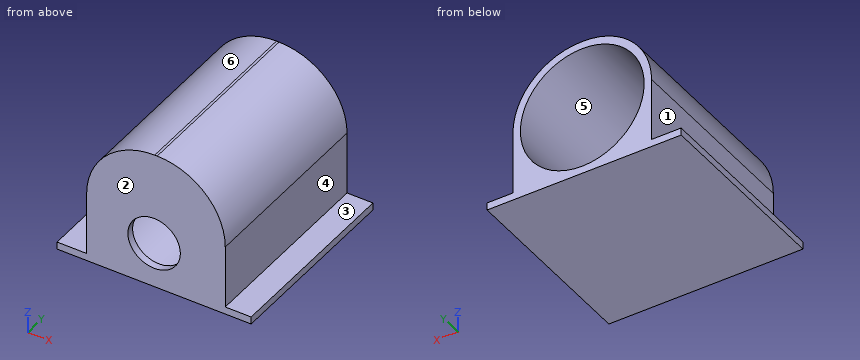
from build123d import *

# Parameters (mm, degrees)
SKETCH018_W     = 52.5
SKETCH018_H     = 2
PAD014_DEPTH    = 51.3
SKETCH028_W     = 37.5
SKETCH028_H     = 51.3
PAD015_DEPTH    = 35.5
FILLET001_R     = 18.416667
SKETCH031_R     = 7.1
POCKET005_DEPTH = 2
SKETCH032_R     = 16.75
POCKET006_DEPTH = 49.3


with BuildPart() as part:
    # Sketch018 → Pad014 (new body)
    with BuildSketch(Plane.XZ):
        with Locations((36.25, 3)):
            Rectangle(SKETCH018_W, SKETCH018_H)
    extrude(amount=-PAD014_DEPTH)

    # Sketch028 (on Face1 of Pad014) → Pad015 (join)
    with BuildSketch(Plane(origin=(0, 0, 4), x_dir=(-1, 0, 0), z_dir=(0, 0, 1))):
        with Locations((-36.75, -25.65)):
            Rectangle(SKETCH028_W, SKETCH028_H)
    extrude(amount=PAD015_DEPTH)

    # Fillet001
    fillet001_edges = [part.edges().sort_by_distance(p)[0] for p in [
        (18, 25.65, 39.5),
        (55.5, 25.65, 39.5),
    ]]
    fillet(fillet001_edges, radius=FILLET001_R)

    # Sketch031 (on Face6 of Pad015) → Pocket005 (cut)
    with BuildSketch(Plane.XZ):
        with Locations((36.25, 14.3)):
            Circle(SKETCH031_R)
    extrude(amount=-POCKET005_DEPTH, mode=Mode.SUBTRACT)

    # Sketch032 (on Face5 of Pocket005) → Pocket006 (cut)
    with BuildSketch(Plane(origin=(0, 51.3, 0), x_dir=(1, 0, 0), z_dir=(0, 1, 0))):
        with Locations((36.75, -20.75)):
            Circle(SKETCH032_R)
    extrude(amount=-POCKET006_DEPTH, mode=Mode.SUBTRACT)


solid = part.part
Here's how the part is built. I have some questions about the finished solid (model axes, mm). Face numbers are marked on the shaded views. A direction names the side the tool comes from. Coordinates: 2 decimals unless noted, no trailing zeros. Loops run counter-clockwise (first coordinate to the right, second up) from the corner with the lowest first, then second, coordinate; pieces in that order, holes last. Notation, with made-up numbers: (76.25, -4) -> (82.25, -4) arc R14 cw to (82.25, 7) -> close; hole circle Ø11 at (-26, 15). An arc over 180 degrees is marked (long way). Use one line per item in the form item = value. Start each with the question number.
(1) On a 3-axis mill with a long thin cutter (end or side, diameter ignored), from which of +Z, -Z, +X, -X, +Y, -Y can I reach the whole of each face in a straight line? I mean the marked faces 1, 2 and 3. Say none if no direction works.
(2) If we section it at C-C (z = 26): Please give me the cut outline in (x, y).
(3) We'd pull the mould along X, two halves only. Please class the marked faces 4, 5 and 6: pulls with the +X half, pulls with the -X half, needs draft (parallel to the pull), parting line crosses it, or undercut.
(4) If we section it at D-D (x = 16.5): Please give me the cut outline in (y, z).
(5) If we section it at A-A (y = 46.5): Please give me the cut outline in (x, z).
(6) Will these pins go through, and if not, where does the flat tip stop? pin 1 (5 mm diameter, centred on y = 34.5, z = 16.5, fed in from -X); pin 2 (3 mm diameter, centred on x = 23, y = 28, fed in from +Z); pin 3 (4 mm diameter, centred on x = 14, y = 37, fed in from +Z).
(7) Please list where these lines run through material, in increasing order: line 1 along Z through (x, y) = (36, 1); line 2 along Z through (x, y) = (36, 15); line 3 along X through (y, z) = (1, 14).
(8) If we section it at B-B (z = 12): Please give me the cut outline in (x, y), then the cut area to 3 significant figures.
Verdict:
q1.face_1 = +Z, -X, +Y, -Y
q1.face_2 = +Z, -Z, +X, -X, -Y
q1.face_3 = +Z, +X, +Y, -Y
q2.outline = (18.67, 0) -> (54.83, 0) -> (54.83, 51.3) -> (52.66, 51.3) -> (52.66, 2) -> (20.84, 2) -> (20.84, 51.3) -> (18.67, 51.3) -> close
q3.face_4 = pulls with the +X half
q3.face_5 = undercut
q3.face_6 = pulls with the -X half
q4.outline = (0, 2) -> (51.3, 2) -> (51.3, 4) -> (0, 4) -> close
q5.outline = (10, 2) -> (62.5, 2) -> (62.5, 4) -> (55.5, 4) -> (55.5, 21.08) arc R18.42 ccw to (37.08, 39.5) -> (36.42, 39.5) arc R18.42 ccw to (18, 21.08) -> (18, 4) -> (10, 4) -> close; hole circle Ø33.5 at (36.75, 20.75)
q6.pin_1 = 18
q6.pin_2 = 35.12
q6.pin_3 = 4
q7.line_1 = 2 to 7.2, 21.4 to 39.5
q7.line_2 = 2 to 4.02, 37.48 to 39.5
q7.line_3 = 18 to 29.16, 43.34 to 55.5
q8.outline = (18, 0) -> (29.53, 0) -> (29.53, 2) -> (22.47, 2) -> (22.47, 51.3) -> (18, 51.3) -> close; (42.97, 0) -> (55.5, 0) -> (55.5, 51.3) -> (51.03, 51.3) -> (51.03, 2) -> (42.97, 2) -> close
q8.area = 489 mm²
